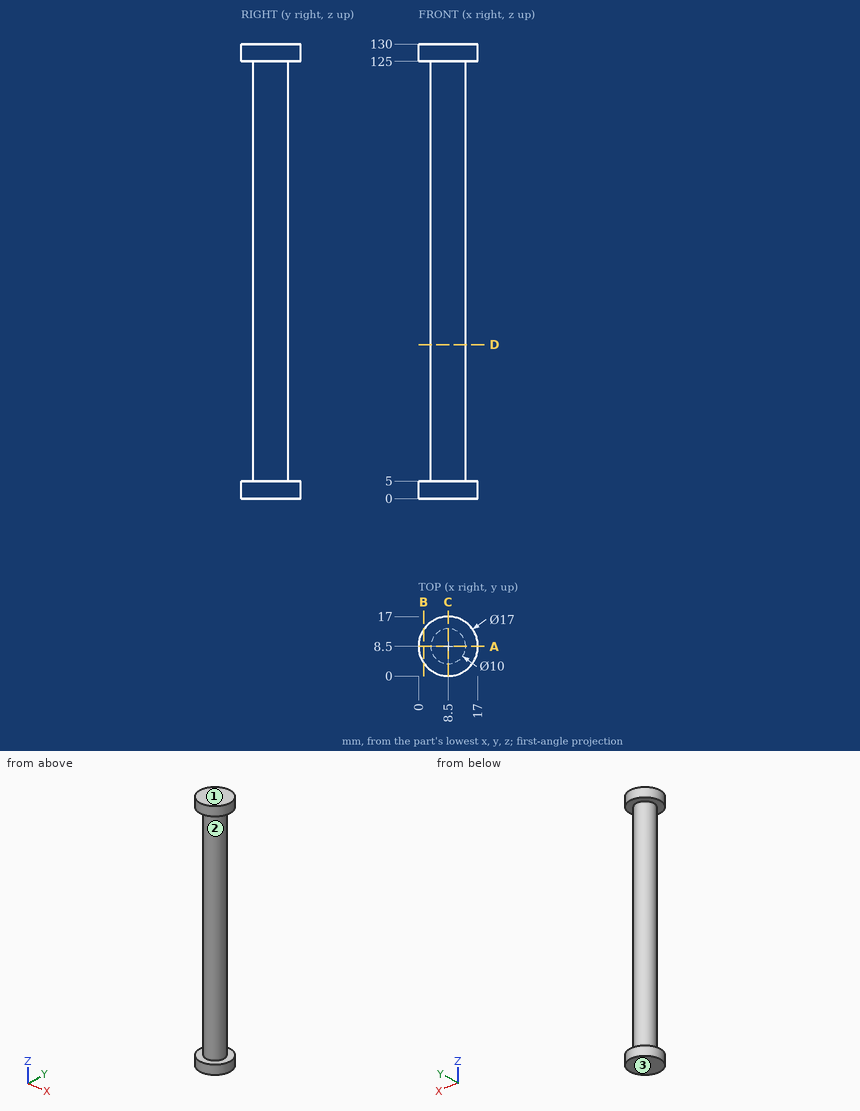
Job drawing, mm, ordinate dimensions from the low corner. One solid piece. Round coordinates to 2 decimals unless told otherwise and drop trailing zeros. Loops run counter-clockwise (first coordinate to the right, second up) from the corner with the lowest first, then second, coordinate; pieces in that order, holes last. Notation, with made-up numbers: M 52.25,-3.75 L 92.25,-3.75 A22 ccw 92.25,9.25 Z; hole C 41,4.25 d9. An arc over 180 degrees is marked long. Answer as CSV lines item,"result".
1. Wall check: probe 1 along Z at (x, y) = (4.25, 3.5); probe 2 along Y at (x, z) = (9, 21). Give the ranges that are in metal, low to high. Write a range as [from, to].
Resolved:
probe 1,"z = [0, 5], [125, 130]"
probe 2,"y = [3.53, 13.47]"
2. Two-plate mould, pull along Z, no slides. Class the marked faces 1, 2 and 3: released by +Z, released by -Z, zero draft, split by the parting line, or undercut.
Resolved:
face 1,"released by +Z"
face 2,"undercut"
face 3,"released by -Z"
3. Cut at D-D on z = 44. Write the cut outline in (x, y).
Resolved:
outline,"C 8.5,8.5 d10"
4. Cut at A-A on y = 8.5. Write the cut outline in (x, z), then the cut area to 3 significant figures.
Resolved:
outline,"M 0,0 L 17,0 L 17,5 L 13.5,5 L 13.5,125 L 17,125 L 17,130 L 0,130 L 0,125 L 3.5,125 L 3.5,5 L 0,5 Z"
area,"1,370 mm²"
5. Flat gauge pins, fed straight in: P1, Ø3, axis at y = 10, z = 52, coming from the -X side; P2, Ø8, axis at x = 7.5, z = 47.5, coming from the +Y side; P3, Ø5, axis at x = 4.5, z = 51, coming from the -Y side. Where does each tip first touch, or does it go through?
Resolved:
P1,"stops at x = 3.5"
P2,"stops at y = 13.5"
P3,"stops at y = 3.73"
6. Cut at B-B on x = 1.5. Write the cut outline in (y, z), then the cut area to 3 significant figures.
Resolved:
outline,"M 3.68,0 L 13.32,0 L 13.32,5 L 3.68,5 Z; M 3.68,125 L 13.32,125 L 13.32,130 L 3.68,130 Z"
area,"96.4 mm²"
